Build history of the part. All positions in model axes, mm. A direction names the side the tool comes from. Coordinates: 2 decimals unless noted, no trailing zeros. Loops run counter-clockwise (first coordinate to the right, second up) from the corner with the lowest first, then second, coordinate; pieces in that order, holes last.
Item 1: Flat gauge pins, fed straight in: pin 1 (6 mm diameter, centred on x = 4, z = 7.5, fed in from +Y); pin 2 (5 mm diameter, centred on x = 19, z = 6.5, fed in from +Y); pin 3 (2 mm diameter, centred on y = -8, z = 6, fed in from +X). Where does each tip first touch, or does it go through?
Item 2: Cut at B-B (z = 8.25). Count the separate pieces of the cut face and the enclosed holes in it, and give its area (3 significant figures).
Item 3: Mould opens along X. For faces 4 (the face through (-13.19, -2.98, 4.93)), 5 (the face through (9.929, 9.174, 4.93)), 6 (the face through (2.99, 13.21, 4.93)) say: released by +X, released by -X, zero draft, split by the parting line, or undercut.
Item 4: Drill centre lines: line 1 along Y through (x, z) = (0, 3.5) (3 decimals); line 2 along Y through (x, z) = (30.75, 7.75); line 3 along X through (y, z) = (13, 7.75). Where is each one in solid material? Low to high.
Item 5: 3-axis set-ups, long thin cutter, end or side, ignore diameter. For faces 1 (the face through (1.423, -12.323, 4.93)), 2 (the face through (9.2, 9.95, 4.93)), 3 (the face through (-4.733, 11.467, 4.93)): which of +Z, -Z, +X, -X, +Y, -Y reach the whole face in a straight line?
Item 6: Cut at A-A (x = 1.5). List the corners of the cut face in (y, z).
from build123d import *

# Parameters (mm, degrees)
SKETCH1_R           = 2
SKETCH1_R_2         = 2.4
BOSS_EXTRUDE1_DEPTH = 10
SKETCH2_R           = 2.4
SKETCH2_R_2         = 1.3
CUT_EXTRUDE1_DEPTH  = 40.007683858


with BuildPart() as part:
    # Sketch1 → Boss-Extrude1 (new body)
    with BuildSketch(Plane.XY):
        with BuildLine():
            Line((0.31, 14.63), (-0.31, 14.63))
            ThreePointArc((-0.31, 14.63), (-0.532517386, 13.523085628), (-0.52, 12.394096377))
            ThreePointArc((-0.52, 12.394096377), (-1.619177414, 12.298873505), (-2.70554676, 12.106363687))
            ThreePointArc((-2.70554676, 12.106363687), (-2.985659813, 13.2001233), (-3.487085624, 14.211728743))
            Line((-3.487085624, 14.211728743), (-4.085959636, 14.051260935))
            ThreePointArc((-4.085959636, 14.051260935), (-4.014404405, 12.924472018), (-3.710109619, 11.837191881))
            ThreePointArc((-3.710109619, 11.837191881), (-4.747187978, 11.460725601), (-5.746714978, 10.993602319))
            ThreePointArc((-5.746714978, 10.993602319), (-6.30036923, 11.977594384), (-7.046532125, 12.824951657))
            Line((-7.046532125, 12.824951657), (-7.583467875, 12.514951657))
            ThreePointArc((-7.583467875, 12.514951657), (-7.222716398, 11.445076999), (-6.647381398, 10.473602319))
            ThreePointArc((-6.647381398, 10.473602319), (-7.551685527, 9.841548186), (-8.396254069, 9.131645121))
            ThreePointArc((-8.396254069, 9.131645121), (-9.185718896, 9.938812205), (-10.125769107, 10.564175311))
            Line((-10.125769107, 10.564175311), (-10.564175311, 10.125769107))
            ThreePointArc((-10.564175311, 10.125769107), (-9.938812205, 9.185718896), (-9.131645121, 8.396254069))
            ThreePointArc((-9.131645121, 8.396254069), (-9.841548186, 7.551685527), (-10.473602319, 6.647381398))
            ThreePointArc((-10.473602319, 6.647381398), (-11.445076999, 7.222716398), (-12.514951657, 7.583467875))
            Line((-12.514951657, 7.583467875), (-12.824951657, 7.046532125))
            ThreePointArc((-12.824951657, 7.046532125), (-11.977594384, 6.30036923), (-10.993602319, 5.746714978))
            ThreePointArc((-10.993602319, 5.746714978), (-11.460725601, 4.747187978), (-11.837191881, 3.710109619))
            ThreePointArc((-11.837191881, 3.710109619), (-12.924472018, 4.014404405), (-14.051260935, 4.085959636))
            Line((-14.051260935, 4.085959636), (-14.211728743, 3.487085624))
            ThreePointArc((-14.211728743, 3.487085624), (-13.2001233, 2.985659813), (-12.106363687, 2.70554676))
            ThreePointArc((-12.106363687, 2.70554676), (-12.298873505, 1.619177414), (-12.394096377, 0.52))
            ThreePointArc((-12.394096377, 0.52), (-13.523085628, 0.532517386), (-14.63, 0.31))
            Line((-14.63, 0.31), (-14.63, -0.31))
            ThreePointArc((-14.63, -0.31), (-13.523085628, -0.532517386), (-12.394096377, -0.52))
            ThreePointArc((-12.394096377, -0.52), (-12.298873505, -1.619177414), (-12.106363687, -2.70554676))
            ThreePointArc((-12.106363687, -2.70554676), (-13.2001233, -2.985659813), (-14.211728743, -3.487085624))
            Line((-14.211728743, -3.487085624), (-14.051260935, -4.085959636))
            ThreePointArc((-14.051260935, -4.085959636), (-12.924472018, -4.014404405), (-11.837191881, -3.710109619))
            ThreePointArc((-11.837191881, -3.710109619), (-11.460725601, -4.747187978), (-10.993602319, -5.746714978))
            ThreePointArc((-10.993602319, -5.746714978), (-11.977594384, -6.30036923), (-12.824951657, -7.046532125))
            Line((-12.824951657, -7.046532125), (-12.514951657, -7.583467875))
            ThreePointArc((-12.514951657, -7.583467875), (-11.445076999, -7.222716398), (-10.473602319, -6.647381398))
            ThreePointArc((-10.473602319, -6.647381398), (1.619177414, -12.298873505), (11.837191881, -3.710109619))
            ThreePointArc((11.837191881, -3.710109619), (12.333238692, -3.879500788), (12.84337176, -4))
            Line((12.84337176, -4), (30.75, -4))
            ThreePointArc((30.75, -4), (34.75, 0), (30.75, 4))
            Line((30.75, 4), (12.84337176, 4))
            ThreePointArc((12.84337176, 4), (12.333238692, 3.879500788), (11.837191881, 3.710109619))
            ThreePointArc((11.837191881, 3.710109619), (11.460725601, 4.747187978), (10.993602319, 5.746714978))
            ThreePointArc((10.993602319, 5.746714978), (11.977594384, 6.30036923), (12.824951657, 7.046532125))
            Line((12.824951657, 7.046532125), (12.514951657, 7.583467875))
            ThreePointArc((12.514951657, 7.583467875), (11.445076999, 7.222716398), (10.473602319, 6.647381398))
            ThreePointArc((10.473602319, 6.647381398), (9.841548186, 7.551685527), (9.131645121, 8.396254069))
            ThreePointArc((9.131645121, 8.396254069), (9.938812205, 9.185718896), (10.564175311, 10.125769107))
            Line((10.564175311, 10.125769107), (10.125769107, 10.564175311))
            ThreePointArc((10.125769107, 10.564175311), (9.185718896, 9.938812205), (8.396254069, 9.131645121))
            ThreePointArc((8.396254069, 9.131645121), (7.551685527, 9.841548186), (6.647381398, 10.473602319))
            ThreePointArc((6.647381398, 10.473602319), (7.222716398, 11.445076999), (7.583467875, 12.514951657))
            Line((7.583467875, 12.514951657), (7.046532125, 12.824951657))
            ThreePointArc((7.046532125, 12.824951657), (6.30036923, 11.977594384), (5.746714978, 10.993602319))
            ThreePointArc((5.746714978, 10.993602319), (4.747187978, 11.460725601), (3.710109619, 11.837191881))
            ThreePointArc((3.710109619, 11.837191881), (4.014404405, 12.924472018), (4.085959636, 14.051260935))
            Line((4.085959636, 14.051260935), (3.487085624, 14.211728743))
            ThreePointArc((3.487085624, 14.211728743), (2.985659813, 13.2001233), (2.70554676, 12.106363687))
            ThreePointArc((2.70554676, 12.106363687), (1.619177414, 12.298873505), (0.52, 12.394096377))
            ThreePointArc((0.52, 12.394096377), (0.532517386, 13.523085628), (0.31, 14.63))
        make_face()
        Circle(SKETCH1_R, mode=Mode.SUBTRACT)
        with Locations((30.75, 0)):
            Circle(SKETCH1_R_2, mode=Mode.SUBTRACT)
    extrude(amount=BOSS_EXTRUDE1_DEPTH)

    # Sketch2 → Cut-Extrude1 (cut, through all)
    with BuildSketch(Plane.XY.offset(10)):
        Circle(SKETCH2_R)
        with Locations((4.5, 0)):
            Circle(SKETCH2_R_2)
        with Locations((-4.5, 0)):
            Circle(SKETCH2_R_2)
    extrude(amount=-CUT_EXTRUDE1_DEPTH, mode=Mode.SUBTRACT)


solid = part.part
Filled sheet:
1. pin 1: stops at y = 14.21
1. pin 2: stops at y = 4
1. pin 3: stops at x = 10.24
2. separate pieces: 1
2. enclosed holes: 4
2. area: 639 mm2
3. face 4: released by -X
3. face 5: released by +X
3. face 6: undercut
4. line 1: y = -12.405 to -2.4, 2.4 to 14.63
4. line 2: y = -4 to -2.4, 2.4 to 4
4. line 3: x = -4.03 to -2.92, -0.56 to 0.56, 2.92 to 4.03
5. face 1: +Z, -Z, -Y
5. face 2: +Z, -Z, +Y
5. face 3: +Z, -Z
6. outline: (-12.31, 0) - (-1.87, 0) - (-1.87, 10) - (-12.31, 10) - close; (1.87, 0) - (12.31, 0) - (12.31, 10) - (1.87, 10) - close
